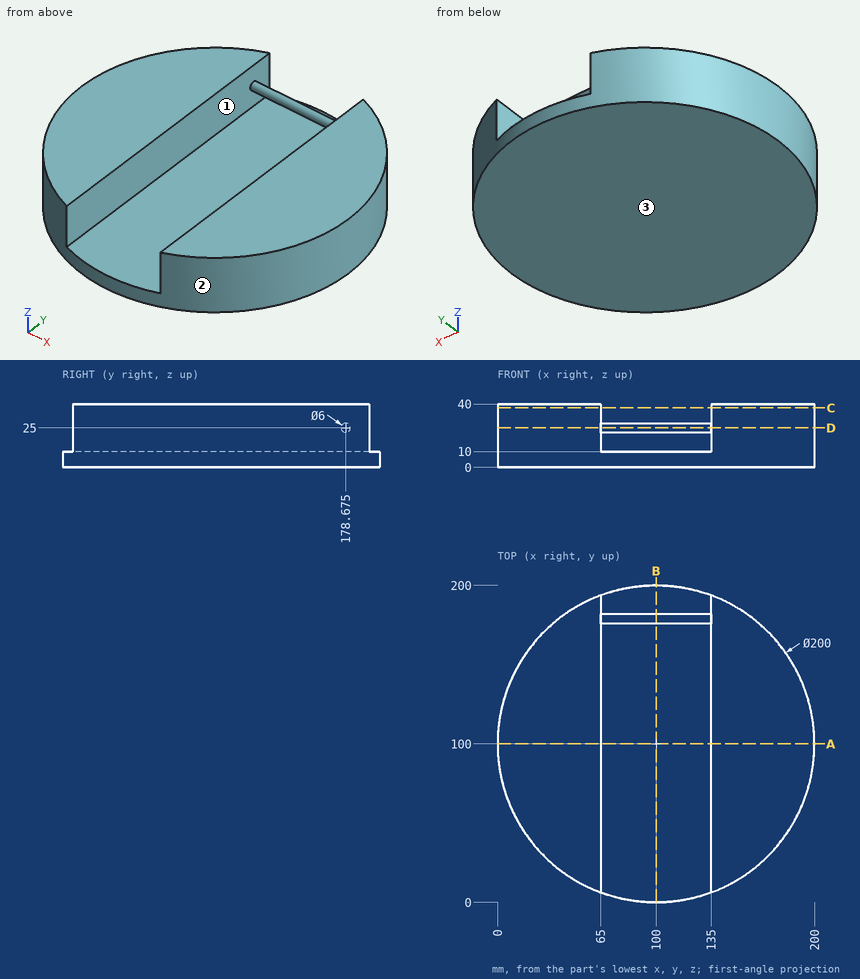
Part print with two shaded views. Sizes in mm from the minimum x, y, z corner. Coordinates: 2 decimals unless noted, no trailing zeros. Write each loop counter-clockwise with the first axis right and the second up, starting at its lowest first coordinate (ties: lowest second). Pieces come first, ordered by that corner, then holes.
(1) Cut at D-D on z = 25. List the corners of the cut face in (x, y) (3 decimals), and give its area (3 significant figures).
(2) Cut at B-B on x = 100. List the corners of the cut face in (y, z) (3 decimals), and give its area (3 significant figures).
(3) Mould opens along X. For the marked faces 1, 2 and 3 say: pulls with the +X half, pulls with the -X half, needs draft (parallel to the pull), parting line crosses it, or undercut.
(4) Cut at C-C on z = 37.5. List the corners of the cut face in (x, y) (3 decimals).
(5) Pin check, flat tips, straight feed: pin 1 Ø4 at (x, z) = (168.5, 16.5) entering from -Y; pin 2 Ø4 at (x, y) = (134, 69) entering from +Z; pin 3 Ø5 at (y, z) = (107.5, 11.5) entering from +X; pin 4 Ø2 at (y, z) = (116.5, 31.5) entering from -X. Stop position of each tip, or through.
(6) Cut at A-A on y = 100. List the corners of the cut face in (x, z).
(7) Drill centre lines: line 1 (Z direction, x = 130.5, y = 155.5); line 2 (X direction, y = 126, z = 15); line 3 (X direction, y = 163.5, z = 20.5). Where is each one in solid material? Low to high.
Working result:
1. outline: (65, 6.325) - (65, 175.675) - (135, 175.675) - (135, 6.325) arc R100 ccw to (135, 193.675) - (135, 181.675) - (65, 181.675) - (65, 193.675) arc R100 ccw to start
1. area: 18,100 mm2
2. outline: (0, 0) - (200, 0) - (200, 10) - (0, 10) - close; circle Ø6 at (178.675, 25)
2. area: 2,030 mm2
3. face 1: undercut
3. face 2: parting line crosses it
3. face 3: needs draft
4. outline: (65, 6.325) - (65, 193.675) arc R100 ccw to start; (135, 6.325) arc R100 ccw to (135, 193.675) - close
5. pin 1: stops at y = 25.32
5. pin 2: stops at z = 40
5. pin 3: stops at x = 199.87
5. pin 4: stops at x = 1.21
6. outline: (0, 0) - (200, 0) - (200, 40) - (135, 40) - (135, 10) - (65, 10) - (65, 40) - (0, 40) - close
7. line 1: z = 0 to 10
7. line 2: x = 3.44 to 65, 135 to 196.56
7. line 3: x = 22.75 to 65, 135 to 177.25
